Could you check a few things on this model? Use its own coordinates, in mm. A direction names the side the tool comes from. Give positions to 0.01 mm unless a question says otherwise; leave off trailing zeros. Order: outer loops, then holes, each group sorted by start corner. A loop starts at its lowest first (then second) coordinate and runs counter-clockwise, first axis right, second up. Notation, with made-up numbers: (-22.75, 77) -> (0.25, 77) arc R27 cw to (0.25, 104) -> close; hole circle Ø11 at (67.5, 34). An arc over 180 degrees is marked (long way). Write each question's results on one line, items separated by ' | '.
```python
from build123d import *

# Parameters (mm, degrees)
F1_DEPTH = 9.525
F2_R     = 9.52499


# Not quite as in the source:
# - a fillet or chamfer is up to 0.001 mm smaller than in the source, because OpenCascade refuses the exact size


with BuildPart() as f1:
    # F0 (on Right) → F1 (new body, symmetric)
    with BuildSketch(Plane.YZ):
        Polygon((-50.8, 6.35), (-50.8, 0), (0, 0), (0, 50.8), (-6.35, 50.8), (-6.35, 6.35), align=None)
    extrude(amount=F1_DEPTH, both=True)

    # F2 (radius 9.525 in the source; OpenCascade refuses exactly that, so slightly less here)
    f2_edges = [f1.edges().sort_by_distance(p)[0] for p in [
        (9.525, -3.175, 50.8),
        (-9.525, -3.175, 50.8),
        (9.525, -50.8, 3.175),
        (-9.525, -50.8, 3.175),
    ]]
    fillet(f2_edges, radius=F2_R)


solid = f1.part
```
Q1. I need wall thicknesses on line 1 along Y through (x, z) = (5.75, 21.5); line 2 along Z through (x, y) = (-5, -30); line 3 along Y through (x, z) = (8.5, 5.5). Which ranges of each line are inside material? Lowest first, please.
Here are the results:
line 1: y = -6.35 to 0 | line 2: z = 0 to 6.35 | line 3: y = -45.57 to 0
Q2. Suppose I cut it at D-D on z = 11. Please give me the cut outline in (x, y) (3 decimals), and give its area (3 significant figures).
Here are the results:
outline: (-9.525, -6.35) -> (9.525, -6.35) -> (9.525, 0) -> (-9.525, 0) -> close | area: 121 mm²
Q3. Suppose I cut it at C-C on y = -35. Please give me the cut outline in (x, z) (3 decimals), and give its area (3 significant figures).
Here are the results:
outline: (-9.525, 0) -> (9.525, 0) -> (9.525, 6.35) -> (-9.525, 6.35) -> close | area: 121 mm²
Q4. I'm going to push flat-ended pins straight in: pin 1 Ø4 at (x, y) = (0.5, -12) entering from +Z; pin 2 Ø5.5 at (x, z) = (-1.5, 30.5) entering from -Y. Where does each tip first touch, or does it pass through?
Here are the results:
pin 1: stops at z = 6.35 | pin 2: stops at y = -6.35
Q5. For faces 1 (the flat face through (0, -28, 6.35)), 2 (the flat face through (0, 0, 25)), which set-ups out of +Z, -Z, +X, -X, +Y, -Y let a thin tool reach every point of the face, with its end or its side?
Here are the results:
face 1: +Z, +X, -X, -Y | face 2: +Z, -Z, +X, -X, +Y
Q6. Suppose I cut it at B-B on x = 6.5. Please give me the cut outline in (y, z), and give its area (3 significant figures).
Here are the results:
outline: (-48.24, 0) -> (0, 0) -> (0, 48.24) -> (-6.35, 48.24) -> (-6.35, 6.35) -> (-48.24, 6.35) -> close | area: 572 mm²
